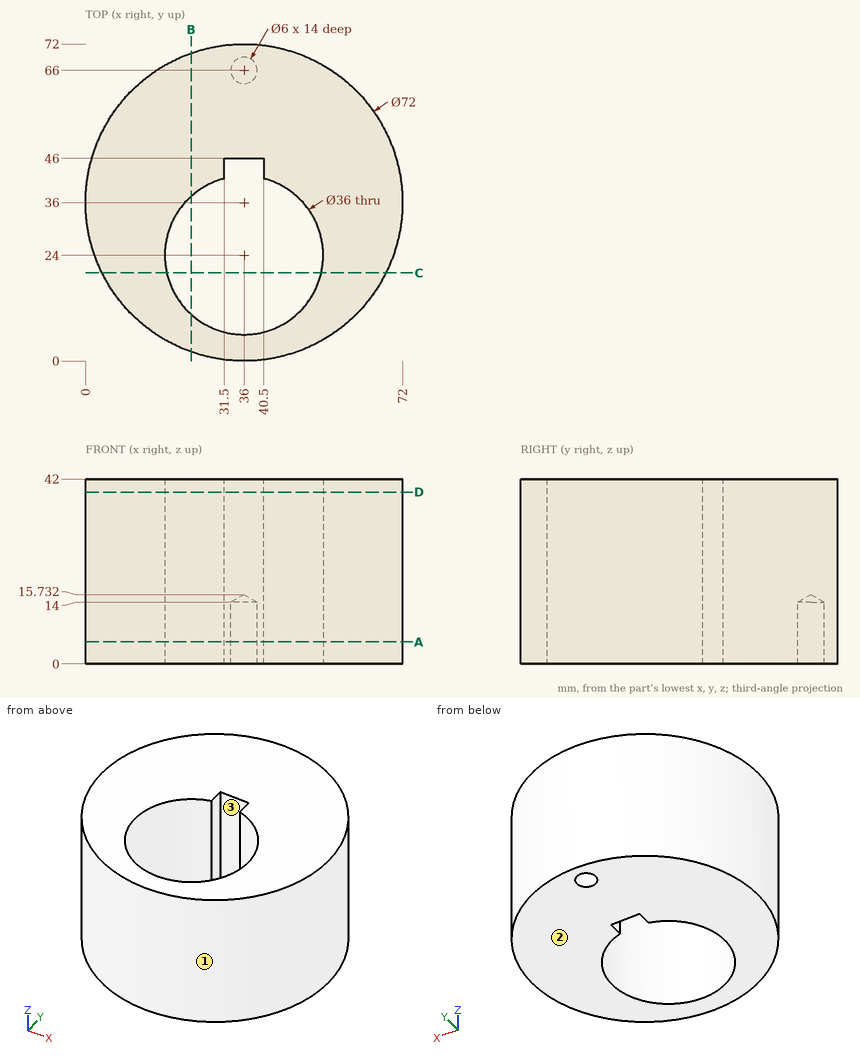
Job drawing, mm, ordinate dimensions from the low corner. One solid piece. Give positions to 0.01 mm unless a question says otherwise; leave off trailing zeros. Loops run counter-clockwise (first coordinate to the right, second up) from the corner with the lowest first, then second, coordinate; pieces in that order, holes last. Notation, with made-up numbers: M -16,23.25 L 34,23.25 A10 ccw 34,35.25 Z; hole C -37.5,26 d5. An arc over 180 degrees is marked long. Put each result on its own line as item: value. Start each with the question number.
1) Saw through at B-B (x = 24). List the corners of the cut face in (y, z).
2) Saw through at C-C (y = 20). List the corners of the cut face in (x, z).
3) Flat gauge pins, fed straight in: pin 1 (4 mm diameter, centred on y = 10.5, z = 26, fed in from -X); pin 2 (1.5 mm diameter, centred on x = 38, z = 4.5, fed in from -Y); pin 3 (4 mm diameter, centred on x = 58, z = 28, fed in from +Y). Where does each tip first touch, or does it go through?
4) Saw through at D-D (z = 39). List the corners of the cut face in (x, y), then the cut area to 3 significant figures.
5) Probe probe 1 along Y at (x, z) = (36, 9); probe 2 along X at (y, z) = (24, 19.5); probe 3 along Y at (x, z) = (23, 28.5). List the from-to ranges inside material, lowest first.
6) Saw through at A-A (z = 5). List the corners of the cut face in (x, y), then the cut area to 3 significant figures.
7) Pull direction X, two halves, no side cores. Call the marked faces 1, 2 and 3: +X half, -X half, draft (parallel to the pull), parting line (faces both ways), or undercut.
Numbers:
1. outline: M 2.06,0 L 10.58,0 L 10.58,42 L 2.06,42 Z; M 37.42,0 L 69.94,0 L 69.94,42 L 37.42,42 Z
2. outline: M 3.75,0 L 18.45,0 L 18.45,42 L 3.75,42 Z; M 53.55,0 L 68.25,0 L 68.25,42 L 53.55,42 Z
3. pin 1: x = 8.73
3. pin 2: y = 0.02
3. pin 3: y = 65.93
4. outline: C 36,36 d72; hole M 31.5,41.43 A18 ccw long 40.5,41.43 L 40.5,46 L 31.5,46 Z
4. area: 3,020 mm^2
5. probe 1: 0 to 6, 46 to 63, 69 to 72
5. probe 2: 2.06 to 18, 54 to 69.94
5. probe 3: 2.43 to 11.55, 36.45 to 69.57
6. outline: C 36,36 d72; hole M 31.5,41.43 A18 ccw long 40.5,41.43 L 40.5,46 L 31.5,46 Z; hole C 36,66 d6
6. area: 2,990 mm^2
7. face 1: parting line
7. face 2: draft
7. face 3: undercut
